Build history of the part. All positions in model axes, mm. Face numbers are marked on the shaded views. A direction names the side the tool comes from. Round coordinates to 2 decimals unless told otherwise and drop trailing zeros. Order: outer loops, then holes, each group sorted by start corner. A loop starts at its lowest first (then second) coordinate and runs counter-clockwise, first axis right, second up. Notation, with made-up numbers: M 83.5,35 L 121.5,35 A5 cw 121.5,40 Z; hole C -38.75,75.5 d5. An arc over 180 degrees is marked long. One line per question, with ' | ' between items. Start each with the question number.
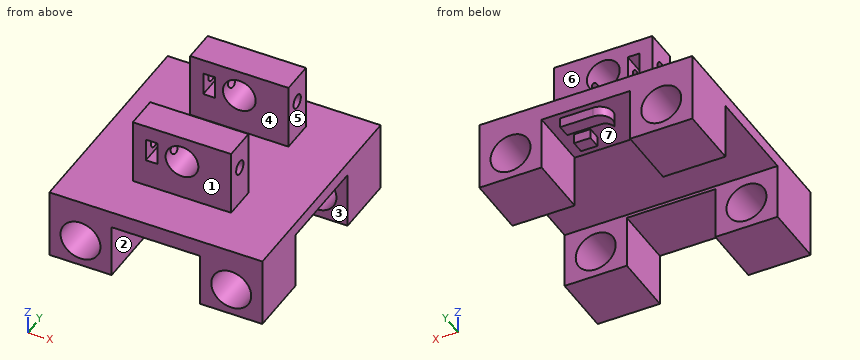
from build123d import *

# Parameters (mm, degrees)
SKETCH1_W           = 19
SKETCH1_H           = 17
SKETCH1_R           = 6.1
BOSS_EXTRUDE1_DEPTH = 68
CUT_EXTRUDE1_REACH  = 80.513
SKETCH3_W           = 65
SKETCH3_H           = 30
SKETCH4_W           = 5
SKETCH4_H           = 4
BOSS_EXTRUDE2_DEPTH = 3
SKETCH5_W           = 30
SKETCH5_H           = 10
BOSS_EXTRUDE3_DEPTH = 20
SKETCH6_R           = 5
CUT_EXTRUDE2_DEPTH  = 75.224322159
SKETCH8_R           = 2.1
CUT_EXTRUDE3_DEPTH  = 90.270655873
CUT_EXTRUDE4_REACH  = 72.386
SKETCH9_W           = 3.5
SKETCH9_H           = 3.5
SKETCH10_W          = 19
SKETCH10_H          = 19
CUT_EXTRUDE5_DEPTH  = 0.7
SKETCH11_W          = 65
SKETCH11_H          = 30
CUT_EXTRUDE6_DEPTH  = 1


with BuildPart() as part:
    # Sketch1 → Boss-Extrude1 (new body)
    # profile 1 of 3: a face of its own
    with BuildSketch(Plane(origin=(0, 0, 0), x_dir=(1, 0, 0), z_dir=(0, 1, 0))):
        with Locations((-23, 0.5)):
            Rectangle(SKETCH1_W, SKETCH1_H)
        with Locations(Location((-23, 0, 0), (0, 0, 270))):
            Circle(SKETCH1_R, mode=Mode.SUBTRACT)
    # profile 2 of 3: a face of its own
    with BuildSketch(Plane(origin=(0, 0, 0), x_dir=(1, 0, 0), z_dir=(0, 1, 0))):
        with Locations((23, 0.5)):
            Rectangle(SKETCH1_W, SKETCH1_H)
        with Locations(Location((23, 0, 0), (0, 0, 270))):
            Circle(SKETCH1_R, mode=Mode.SUBTRACT)
    # profile 3 of 3: a face of its own
    with BuildSketch(Plane(origin=(0, 0, 0), x_dir=(1, 0, 0), z_dir=(0, 1, 0))):
        Polygon((-13.5, -8), (13.5, -8), (32.5, -8), (32.5, -13), (-32.5, -13), (-32.5, -8), align=None)
    extrude(amount=BOSS_EXTRUDE1_DEPTH)

    # Cut-Extrude1: up to this face of the body (flat: up to its plane)
    cut_extrude1_end = Plane(part.part.faces().sort_by_distance((0, 34, 8))[0])
    # Sketch3 → Cut-Extrude1 (cut, up to the picked face)
    with BuildSketch(Plane(origin=(0, 0, -9), x_dir=(-1, 0, 0), z_dir=(0, 0, -1)), mode=Mode.PRIVATE) as cut_extrude1_sk1:
        with Locations((0, 34)):
            Rectangle(SKETCH3_W, SKETCH3_H)
    cut_extrude1_tool1 = split(extrude(cut_extrude1_sk1.sketch, amount=-CUT_EXTRUDE1_REACH, mode=Mode.PRIVATE), bisect_by=cut_extrude1_end, keep=Keep.BOTH, mode=Mode.PRIVATE)
    add(cut_extrude1_tool1.solids().sort_by(Axis((0, 34, -9), (0, 0, 1)))[0], mode=Mode.SUBTRACT)

    # Sketch4 → Boss-Extrude2 (add)
    with BuildSketch(Plane(origin=(0, 0, 8), x_dir=(-1, 0, 0), z_dir=(0, 0, -1))):
        with BuildLine():
            ThreePointArc((4.191236083, 59.518146972), (4.82097308, 63.804174702), (1.17903595, 66.15))
            Line((1.17903595, 66.15), (-8.82096405, 66.15))
            Line((-8.82096405, 66.15), (-8.82096405, 62.15))
            Line((-8.82096405, 62.15), (1.17903595, 62.15))
            ThreePointArc((1.17903595, 62.15), (3.230210626, 61.45792056), (4.191236083, 59.518146972))
        make_face()
        with Locations((-6.32096405, 56.15)):
            Rectangle(SKETCH4_W, SKETCH4_H)
    extrude(amount=BOSS_EXTRUDE2_DEPTH)

    # Sketch5 → Boss-Extrude3 (add)
    with BuildSketch(Plane.XY.offset(13)):
        with Locations((0, 20)):
            Rectangle(SKETCH5_W, SKETCH5_H)
        with Locations((0, 53)):
            Rectangle(SKETCH5_W, SKETCH5_H)
    extrude(amount=BOSS_EXTRUDE3_DEPTH)

    # Sketch6 → Cut-Extrude2 (cut, through all)
    with BuildSketch(Plane(origin=(0, 58, 0), x_dir=(1, 0, 0), z_dir=(0, 1, 0))):
        with Locations(Location((0, -25, 0), (0, 0, 270))):
            Circle(SKETCH6_R)
    extrude(amount=-CUT_EXTRUDE2_DEPTH, mode=Mode.SUBTRACT)

    # Sketch8 → Cut-Extrude3 (cut, through all)
    with BuildSketch(Plane.ZY.offset(15)):
        with Locations((25, 20)):
            Circle(SKETCH8_R)
        with Locations((25, 53)):
            Circle(SKETCH8_R)
    extrude(amount=-CUT_EXTRUDE3_DEPTH, mode=Mode.SUBTRACT)

    # Cut-Extrude4: up to this face of the body (flat: up to its plane)
    cut_extrude4_end = Plane(part.part.faces().sort_by_distance((14.639444872, 58, 23))[0])
    # Sketch9 → Cut-Extrude4 (cut, up to the picked face)
    with BuildSketch(Plane.XZ.offset(-15), mode=Mode.PRIVATE) as cut_extrude4_sk1:
        with Locations((-9.25, 23.25)):
            Rectangle(SKETCH9_W, SKETCH9_H)
    cut_extrude4_tool1 = split(extrude(cut_extrude4_sk1.sketch, amount=-CUT_EXTRUDE4_REACH, mode=Mode.PRIVATE), bisect_by=cut_extrude4_end, keep=Keep.BOTH, mode=Mode.PRIVATE)
    # Sketch9 → Cut-Extrude4 (cut, up to the picked face)
    with BuildSketch(Plane.XZ.offset(-15), mode=Mode.PRIVATE) as cut_extrude4_sk2:
        with Locations((-9.25, 26.75)):
            Rectangle(SKETCH9_W, SKETCH9_H)
    cut_extrude4_tool2 = split(extrude(cut_extrude4_sk2.sketch, amount=-CUT_EXTRUDE4_REACH, mode=Mode.PRIVATE), bisect_by=cut_extrude4_end, keep=Keep.BOTH, mode=Mode.PRIVATE)
    add(cut_extrude4_tool1.solids().sort_by(Axis((-9.25, 15, 23.25), (0, 1, 0)))[0], mode=Mode.SUBTRACT)
    add(cut_extrude4_tool2.solids().sort_by(Axis((-9.25, 15, 26.75), (0, 1, 0)))[0], mode=Mode.SUBTRACT)

    # Sketch10 → Cut-Extrude5 (cut)
    with BuildSketch(Plane(origin=(0, 0, -9), x_dir=(-1, 0, 0), z_dir=(0, 0, -1))):
        with Locations((23, 9.5)):
            Rectangle(SKETCH10_W, SKETCH10_H)
        with Locations((-23, 9.5)):
            Rectangle(SKETCH10_W, SKETCH10_H)
        with Locations((23, 58.5)):
            Rectangle(SKETCH10_W, SKETCH10_H)
        with Locations((-23, 58.5)):
            Rectangle(SKETCH10_W, SKETCH10_H)
    extrude(amount=-CUT_EXTRUDE5_DEPTH, mode=Mode.SUBTRACT)

    # Sketch11 → Cut-Extrude6 (cut)
    with BuildSketch(Plane(origin=(0, 0, 8), x_dir=(-1, 0, 0), z_dir=(0, 0, -1))):
        with Locations((0, 34)):
            Rectangle(SKETCH11_W, SKETCH11_H)
    extrude(amount=-CUT_EXTRUDE6_DEPTH, mode=Mode.SUBTRACT)


solid = part.part
Item 1: Wall check: line 1 along Y through (x, z) = (-12.7, 25); line 2 along X through (y, z) = (12, 0); line 3 along Y through (x, z) = (6, 28.5). Give the ranges that are in metal, low to high. Write a range as [from, to].
Item 2: Cut at B-B on z = 18. Write the cut outline in (x, y), then the cut area to 3 significant figures.
Item 3: Cut at C-C on y = 13. Write the cut outline in (x, z), then the cut area to 3 significant figures.
Item 4: Flat gauge pins, fed straight in: pin 1 (8 mm diameter, centred on y = 54, z = 27, fed in from +X); pin 2 (1 mm diameter, centred on x = -6.5, z = 19.5, fed in from +Y); pin 3 (5.5 mm diameter, centred on x = 3, y = 63.5, fed in from -Z). Where does each tip first touch, or does it go through?
Item 5: Tool access for the marked faces 1, 2, 3 and 4: list every direction of +Z, -Z, +X, -X, +Y, -Y with a clear straight run to the whole face (end or side of a thin tool).
Item 6: Cut at D-D on x = 0. Write the cut outline in (y, z), then the cut area to 3 significant figures.
Item 7: Cut at A-A on y = 53. Count the separate pieces of the cut face and the enclosed holes in it, then the cut area to 3 significant figures.
Item 8: Two-plate mould, pull along X, no slides. Class the marked faces 5, 6 and 7: +X half, -X half, draft (parallel to the pull), parting line (faces both ways), or undercut.
Results found:
1) line 1: y = [15, 17.9], [22.1, 25], [48, 50.9], [55.1, 58] | line 2: x = [-32.5, -29.1], [-16.9, -13.5], [13.5, 16.9], [29.1, 32.5] | line 3: y = [15, 25], [48, 58]
2) outline: M -15,15 L 15,15 L 15,25 L -15,25 Z; M -15,48 L 15,48 L 15,58 L -15,58 Z | area: 600 mm^2
3) outline: M -32.5,-8.3 L -13.5,-8.3 L -13.5,8 L 13.5,8 L 13.5,-8.3 L 32.5,-8.3 L 32.5,13 L -32.5,13 Z; hole C -23,0 d12.2; hole C 23,0 d12.2 | area: 711 mm^2
4) pin 1: stops at x = 15 | pin 2: stops at y = 58 | pin 3: stops at z = 5
5) face 1: +Z, +X, -X, -Y | face 2: -Z, +Y, -Y | face 3: -Z, +X, -X | face 4: +Z, +X, -X
6) outline: M 0,8 L 19,8 L 19,9 L 49,9 L 49,8 L 62.15,8 L 62.15,5 L 66.15,5 L 66.15,8 L 68,8 L 68,13 L 58,13 L 58,20 L 48,20 L 48,13 L 25,13 L 25,20 L 15,20 L 15,13 L 0,13 Z; M 15,30 L 25,30 L 25,33 L 15,33 Z; M 48,30 L 58,30 L 58,33 L 48,33 Z | area: 522 mm^2
7) separate pieces: 2 | enclosed holes: 2 | area: 1,140 mm^2
8) face 5: +X half | face 6: draft | face 7: undercut
